```python
from build123d import *

# Parameters (mm, degrees)
SKETCH1_W           = 50.8
SKETCH1_H           = 53.975
BOSS_EXTRUDE1_DEPTH = 3.175
SKETCH2_R           = 2.032
CUT_EXTRUDE1_DEPTH  = 38.196314082
FILLET1_R           = 2.54
FILLET2_R           = 6.35


with BuildPart() as part:
    # Sketch1 → Boss-Extrude1 (new body)
    with BuildSketch(Plane(origin=(0, 0, 0), x_dir=(1, 0, 0), z_dir=(0, 1, 0))):
        Rectangle(SKETCH1_W, SKETCH1_H)
    extrude(amount=BOSS_EXTRUDE1_DEPTH)

    # Sketch2 → Cut-Extrude1 (cut, through all)
    with BuildSketch(Plane(origin=(0, 0, 0), x_dir=(-1, 0, 0), z_dir=(0, -1, 0))):
        with Locations(Location((-19.05, -22.225, 0), (0, 0, 90))):
            Circle(SKETCH2_R)
        with Locations(Location((19.05, -22.225, 0), (0, 0, 90))):
            Circle(SKETCH2_R)
    extrude(amount=-CUT_EXTRUDE1_DEPTH, mode=Mode.SUBTRACT)

    # Fillet1
    fillet1_edges = [part.edges().sort_by_distance(p)[0] for p in [
        (25.4, 1.5875, 26.9875),
        (-25.4, 1.5875, 26.9875),
    ]]
    fillet(fillet1_edges, radius=FILLET1_R)

    # Fillet2
    fillet2_edges = [part.edges().sort_by_distance(p)[0] for p in [
        (-25.4, 1.5875, -26.9875),
        (25.4, 1.5875, -26.9875),
    ]]
    fillet(fillet2_edges, radius=FILLET2_R)


solid = part.part
```
Geometry check sheet. Reference: the model listing, model coordinates, mm. Coordinates: 2 decimals unless noted, no trailing zeros.
Item 1: Thickness scan on line 1 (X direction, y = 1.1, z = 23.5); line 2 (X direction, y = 1.35, z = -22); line 3 (X direction, y = 1.2, z = -22.5). Record the ranges inside material, lowest first.
Item 2: Sectioned sample at A-A, the plane y = 1.45. Count the separate pieces of the cut face and the enclosed holes in it, then the cut area to 3 significant figures.
Item 3: Release check for a two-part mould opening along X. For faces 1 (the face through (-18.4, 1.6, 20.3)), 2 (the face through (-23.59, 1.61, -25.08)), 3 (the face through (0, 2, -26.988)), 4 (the face through (19.7, 1.6, 20.3)) record: released by +X, released by -X, zero draft, split by the parting line, or undercut.
Item 4: Go/stop test with a flat-tipped pin: pin 1 Ø1 at (x, y) = (-20, 1.5) entering from -Z. Record where the tip stops, or that it passes through.
Check result:
1. line 1: x = -25.4 to -20.63, -17.47 to 17.47, 20.63 to 25.4
1. line 2: x = -25.25 to 25.25
1. line 3: x = -25.12 to 25.12
2. separate pieces: 1
2. enclosed holes: 2
2. area: 2,700 mm2
3. face 1: undercut
3. face 2: released by -X
3. face 3: zero draft
3. face 4: undercut
4. pin 1: stops at z = -26.97
